Autodesk Inventor part; units mm, degrees
ref_plane "YZ Plane" through (0, 0, 0) normal (1, 0, 0) x (0, 1, 0)
ref_plane "XZ Plane" through (0, 0, 0) normal (0, 1, 0) x (-1, 0, 0)
ref_plane "XY Plane" through (0, 0, 0) normal (0, 0, 1) x (1, 0, 0)
sketch "Boceto1" plane through (0, 0, 0) normal (0, 0, 1) x (1, 0, 0)
  line L0 (0, 100) -> (0, 0)
  line L1 (-100, 25) -> (-100, 75)
  line L2 (-75, 0) -> (-75, -3)
  line L3 (-75, -3) -> (-25, -3)
  line L4 (-25, -3) -> (-25, 0)
  line L5 (0, 0) -> (-25, 0)
  line L6 (-103, 100) -> (-103, 75)
  line L7 (-103, 75) -> (-100, 75)
  line L8 (-103, 0) -> (-103, 25)
  line L9 (-103, 25) -> (-100, 25)
  line L10 (-103, 0) -> (-75, 0)
  line L11 (-75, 100) -> (-75, 103)
  line L12 (-75, 103) -> (-25, 103)
  line L13 (-25, 103) -> (-25, 100)
  line L14 (0, 100) -> (-25, 100)
  line L15 (-75, 100) -> (-103, 100)
  line L16 (-75, 66.9731) -> (-66.9731, 75)
  line L17 (-75, 66.9731) -> (-63.6482, 66.9731) construction
  line L18 (-75, 59.902) -> (-59.902, 75)
  line L19 (-75, 52.8309) -> (-52.8309, 75)
  line L20 (-75, 45.7599) -> (-45.7599, 75)
  line L21 (-75, 38.6888) -> (-38.6888, 75)
  line L22 (-75, 31.6177) -> (-31.6177, 75)
  line L23 (-74.5467, 25) -> (-25, 74.5467)
  line L24 (-67.4756, 25) -> (-25, 67.4756)
  line L25 (-60.4045, 25) -> (-25, 60.4045)
  line L26 (-53.3335, 25) -> (-25, 53.3335)
  line L27 (-46.2624, 25) -> (-25, 46.2624)
  line L28 (-39.1913, 25) -> (-25, 39.1913)
  line L29 (-32.1203, 25) -> (-25, 32.1203)
  line L30 (-66.9731, 75) -> (-59.902, 75)
  line L31 (-75, 59.902) -> (-75, 66.9731)
  line L32 (-75, 31.6177) -> (-75, 38.6888)
  line L33 (-75, 45.7599) -> (-75, 52.8309)
  line L34 (-52.8309, 75) -> (-45.7599, 75)
  line L35 (-38.6888, 75) -> (-31.6177, 75)
  line L36 (-67.4756, 25) -> (-74.5467, 25)
  line L37 (-25, 74.5467) -> (-25, 67.4756)
  line L38 (-25, 60.4045) -> (-25, 53.3335)
  line L39 (-53.3335, 25) -> (-60.4045, 25)
  line L40 (-25, 25) -> (-32.1203, 25)
  line L41 (-39.1913, 25) -> (-46.2624, 25)
  line L42 (-25, 46.2624) -> (-25, 39.1913)
  line L43 (-25, 32.1203) -> (-25, 25)
  dimension "d1" = 100
  dimension "d4" = 50
  dimension "d5" = 25
  dimension "d7" = 25
  dimension "d8" = 25
  dimension "d9" = 3
  dimension "d10" = 3
  dimension "d11" = 100
  dimension "d13" = 50
  dimension "d14" = 3
  dimension "d15" = 45
  dimension "d16" = 5
  dimension "d17" = 5
  dimension "d18" = 5
  dimension "d19" = 5
  dimension "d20" = 5
  dimension "d21" = 5
  dimension "d22" = 5
  dimension "d25" = 5
  dimension "d26" = 5
  dimension "d27" = 5
  dimension "d28" = 5
  dimension "d29" = 5
  dimension "d30" = 25
  dimension "d31" = 25
  dimension "d32" = 11.3518
extrude "Extrusión1" add sketch "Boceto1" along normal blind 3
properties part number "Control lateral"
Design review of the part built by this model. Coordinates are the model's own, in mm. A direction names the side the tool comes from. Give positions to 0.01 mm unless a question says otherwise; leave off trailing zeros. Loops run counter-clockwise (first coordinate to the right, second up) from the corner with the lowest first, then second, coordinate; pieces in that order, holes last. Notation, with made-up numbers: M 27,-22 L 82,-22 A5 ccw 82,-16 Z; hole C -36.5,3 d8. An arc over 180 degrees is marked long. Answer as a JSON object with one key per item and string values.
Item 1: We need section B-B (y = 34). State the section outline as (x, z) points.
Output values:
{"outline": "M -100,0 L -75,0 L -75,3 L -100,3 Z; M -72.62,0 L -65.55,0 L -65.55,3 L -72.62,3 Z; M -58.48,0 L -51.4,0 L -51.4,3 L -58.48,3 Z; M -44.33,0 L -37.26,0 L -37.26,3 L -44.33,3 Z; M -30.19,0 L 0,0 L 0,3 L -30.19,3 Z"}
Item 2: We need section A-A (x = -72). State the section outline as (y, z) points, and give its area (3 significant figures).
Output values:
{"outline": "M -3,0 L 25,0 L 25,3 L -3,3 Z; M 27.55,0 L 34.62,0 L 34.62,3 L 27.55,3 Z; M 41.69,0 L 48.76,0 L 48.76,3 L 41.69,3 Z; M 55.83,0 L 62.9,0 L 62.9,3 L 55.83,3 Z; M 69.97,0 L 103,0 L 103,3 L 69.97,3 Z", "area": "247 mm2"}
Item 3: For P1, Ø1.5, axis at y = -2, z = 1.5, coming from the -X side; P2, Ø1.5, axis at y = 72, z = 2, coming from the -X side; P3, Ø1.5, axis at x = -101.5, z = 1.5, coming from the +Y side, all flat-tipped, find the tip position at first contact; note any pin that passes through.
Output values:
{"P1": "stops at x = -75", "P2": "stops at x = -100", "P3": "stops at y = 100"}
Item 4: Mouldability with a two-part tool opening along X and no side actions: class faces 5 (the face through (0, 51, 1)), 6 (the face through (-71, 25, 1)), 7 (the face through (-75, 101, 1)), 8 (the face through (-89, 0, 1)) as pulls with the +X half, pulls with the -X half, needs draft (parallel to the pull), parting line crosses it, or undercut.
Output values:
{"face 5": "pulls with the +X half", "face 6": "undercut", "face 7": "pulls with the -X half", "face 8": "needs draft"}
Item 5: Wall thickness on line 1 along Y through (x, z) = (-59.5, 2.85); line 2 along X through (y, z) = (57, 0.3); line 3 along Y through (x, z) = (-50, 0.7): over which ranges is each line inside the solid? List them lowest first.
Output values:
{"line 1": "y = -3 to 25, 25.9 to 32.98, 40.05 to 47.12, 54.19 to 61.26, 68.33 to 103", "line 2": "x = -100 to -70.83, -63.76 to -56.69, -49.62 to -42.55, -35.48 to -28.4, -25 to 0", "line 3": "y = -3 to 28.33, 35.4 to 42.48, 49.55 to 56.62, 63.69 to 70.76, 75 to 103"}
Item 6: We need section C-C (z = 2.3). Count the separate pieces of the cut face and the enclosed holes in it, and give its area (3 significant figures).
Output values:
{"separate pieces": "1", "enclosed holes": "7", "area": "9,200 mm2"}
Item 7: Machinability: for faces 1 (the face through (-32.19, 32, 1.48)), 2 (the face through (-12, 0, 1)), 3 (the face through (-102, 75, 1)), 4 (the face through (-89, 100, 1)), which of the approach directions +Z, -Z, +X, -X, +Y, -Y give a long, thin tool a straight path to every point of the face, cutting with its end or side? Answer none if there is none.
Output values:
{"face 1": "+Z, -Z", "face 2": "+Z, -Z, +X, -Y", "face 3": "+Z, -Z, -X", "face 4": "+Z, -Z, -X, +Y"}
